Work out the finished part from the listing and answer in its coordinate system (mm). Face numbers are marked on the shaded views. A direction names the side the tool comes from. Coordinates: 2 decimals unless noted, no trailing zeros. Write each loop counter-clockwise with the first axis right and the second up, starting at its lowest first coordinate (ties: lowest second). Pieces come first, ordered by that corner, then holes. Notation, with made-up numbers: (40.25, 40) - (74.25, 40) arc R16 cw to (74.25, 65) - close; hole circle Ø7 at (62, -33.75). An arc over 180 degrees is marked (long way). Use CSV: the item, a comma, the result in double quotes. Start each with the question number.
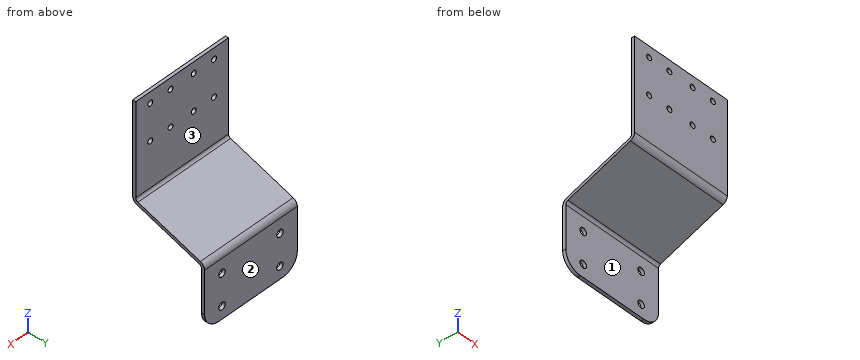
from build123d import *

# Parameters (mm, degrees)
BASE_FLANGE1_DEPTH   = 32
M3_CLEARANCE_HOLE1_D = 3.4
M4_CLEARANCE_HOLE1_D = 4.5
FILLET1_R            = 10


# Sheet-metal steps are written as plain solids
with BuildPart() as part:
    # Sketch1 → Base-Flange1 (new, symmetric)
    with BuildSketch(Plane(origin=(0, 0, 0), x_dir=(0, 0, -1), z_dir=(1, 0, 0))):
        with BuildLine():
            Line((0, 0), (58.568792855, 0))
            ThreePointArc((58.568792855, 0), (59.732688101, 0.373547463), (60.461813231, 1.354652144))
            Line((60.461813231, 1.354652144), (74.076373538, 41.290695711))
            ThreePointArc((74.076373538, 41.290695711), (75.534623798, 43.252905074), (77.862414291, 44))
            Line((77.862414291, 44), (115, 44))
            Line((115, 44), (115, 42))
            Line((115, 42), (77.862414291, 42))
            ThreePointArc((77.862414291, 42), (76.698519044, 41.626452537), (75.969393914, 40.645347856))
            Line((75.969393914, 40.645347856), (62.354833607, 0.709304289))
            ThreePointArc((62.354833607, 0.709304289), (60.896583347, -1.252905074), (58.568792855, -2))
            Line((58.568792855, -2), (0, -2))
            Line((0, -2), (0, 0))
        make_face()
    extrude(amount=BASE_FLANGE1_DEPTH, both=True)

    # M3 Clearance Hole1 (through all)
    with Locations(Plane(origin=(0, 0, 0), x_dir=(1, 0, 0), z_dir=(0, 1, 0))):
        with Locations((-22, 30), (-22, 7), (-8, 7), (-8, 30), (8, 30), (8, 7), (22, 7), (22, 30)):
            Hole(M3_CLEARANCE_HOLE1_D / 2)

    # M4 Clearance Hole1 (through all)
    with Locations(Plane(origin=(0, 44, 0), x_dir=(1, 0, 0), z_dir=(0, 1, 0))):
        with Locations((-20, 107), (-20, 87), (20, 87), (20, 107)):
            Hole(M4_CLEARANCE_HOLE1_D / 2)

    # Fillet1
    fillet1_edges = [part.edges().sort_by_distance(p)[0] for p in [
        (-32, 43, -115),
        (32, 43, -115),
    ]]
    fillet(fillet1_edges, radius=FILLET1_R)


solid = part.part
Item 1: Each of these flat-tipped pins is pushed along its axis until it touches: pin 1 (4 mm diameter, centred on x = -9.5, y = 30, fed in from -Z); pin 2 (1.5 mm diameter, centred on x = 22, z = -35, fed in from +Y); pin 3 (11 mm diameter, centred on x = 10.5, z = -99, fed in from -Y). Where does it stop, or does it pass through?
Item 2: Straight lines are drawn through the part: probe 1 along X at (y, z) = (-1.4, -30); probe 2 along Z at (x, y) = (20, 43); probe 3 along Z at (x, y) = (8, -0.8). For each, find the intervals that lie inside material, in ascending order. Write a range as [from, to].
Item 3: Which of the six approach directions +Z, -Z, +X, -X, +Y, -Y give full straight-line access (tool end or side, diameter ignored) to the marked faces 1, 2 and 3?
Item 4: A cutting plane is placed at A-A (z = -87). Determine the outline of the cut face in (x, y), then the cut area to 3 significant figures.
Item 5: A cutting plane is placed at B-B (x = 8). Determine the outline of the cut face in (y, z).
Item 6: A cutting plane is placed at C-C (x = -4.5). Determine the outline of the cut face in (y, z), then the cut area to 3 significant figures.
Item 7: A cutting plane is placed at D-D (z = -7). Determine the outline of the cut face in (x, y).
Calculated:
1,pin 1,"stops at z = -73.02"
1,pin 2,"stops at y = 0"
1,pin 3,"stops at y = 42"
2,probe 1,"x = [-32, -23.7], [-20.3, -9.7], [-6.3, 6.3], [9.7, 20.3], [23.7, 32]"
2,probe 2,"z = [-115, -109.25], [-104.75, -89.25], [-84.75, -75.22]"
2,probe 3,"z = [-61.43, -31.7], [-28.3, -8.7], [-5.3, 0]"
3,face 1,"-Z, +X, -X, -Y"
3,face 2,"+Z, -Z, +X, -X, +Y"
3,face 3,"+Z, +X, -X, +Y"
4,outline,"(-32, 42) - (-22.25, 42) - (-22.25, 44) - (-32, 44) - close; (-17.75, 42) - (17.75, 42) - (17.75, 44) - (-17.75, 44) - close; (22.25, 42) - (32, 42) - (32, 44) - (22.25, 44) - close"
4,area,"110 mm²"
5,outline,"(-2, -58.57) arc R4 ccw to (0.71, -62.35) - (40.65, -75.97) arc R2 cw to (42, -77.86) - (42, -115) - (44, -115) - (44, -77.86) arc R4 ccw to (41.29, -74.08) - (1.35, -60.46) arc R2 cw to (0, -58.57) - (0, -31.7) - (-2, -31.7) - close; (-2, -28.3) - (0, -28.3) - (0, -8.7) - (-2, -8.7) - close; (-2, -5.3) - (0, -5.3) - (0, 0) - (-2, 0) - close"
6,outline,"(-2, -58.57) arc R4 ccw to (0.71, -62.35) - (40.65, -75.97) arc R2 cw to (42, -77.86) - (42, -115) - (44, -115) - (44, -77.86) arc R4 ccw to (41.29, -74.08) - (1.35, -60.46) arc R2 cw to (0, -58.57) - (0, 0) - (-2, 0) - close"
6,area,"291 mm²"
7,outline,"(-32, -2) - (-23.7, -2) - (-23.7, 0) - (-32, 0) - close; (-20.3, -2) - (-9.7, -2) - (-9.7, 0) - (-20.3, 0) - close; (-6.3, -2) - (6.3, -2) - (6.3, 0) - (-6.3, 0) - close; (9.7, -2) - (20.3, -2) - (20.3, 0) - (9.7, 0) - close; (23.7, -2) - (32, -2) - (32, 0) - (23.7, 0) - close"
